The drawing under review shows one solid part. Ordinate dimensions are in mm from its lowest x, y, z. A direction names the side the tool comes from. Give positions to 0.01 mm unless a question says otherwise; leave off trailing zeros. Write each loop counter-clockwise with the first axis right and the second up, starting at its lowest first coordinate (ties: lowest second). Pieces come first, ordered by that corner, then holes.
Q1. We need section D-D (y = 16.75). Write out the cut boundary in (x, z).
Q2. Machinability: for the marked faces 1, 2, 3, 4 and 5, which of the approach directions +Z, -Z, +X, -X, +Y, -Y give a long, thin tool a straight path to every point of the face, cutting with its end or side? Answer none if there is none.
Q3. For line 1 (X direction, y = 4, z = 7.5); line 2 (Z direction, x = 37, y = 14); line 3 (Z direction, x = 5, y = 5.25), list the stretches that pass through material, from the lowest coordinate up.
Q4. We need section C-C (x = 6). Write out the cut boundary in (y, z).
Q5. We need section A-A (z = 17.5). Write out the cut boundary in (x, y).
Q6. Insertion check: P1, Ø5.5, axis at x = 36, z = 19, coming from the -Y side; P2, Ø5, axis at x = 7, z = 7.5, coming from the -Y side; P3, Ø1.5, axis at y = 2, z = 6, coming from the +X side; P4, Ø0.6, axis at y = 1, z = 15, coming from the +X side. Each pin has a flat end and moves straight along its axis. Give the tip position at first contact, or say it passes through.
Q7. We need section B-B (x = 37). Write out the cut boundary in (y, z).
Q8. Mouldability with a two-part tool opening along Z and no side actions: class the marked faces 6, 7, 8 and 9 as released by +Z, released by -Z, zero draft, split by the parting line, or undercut.
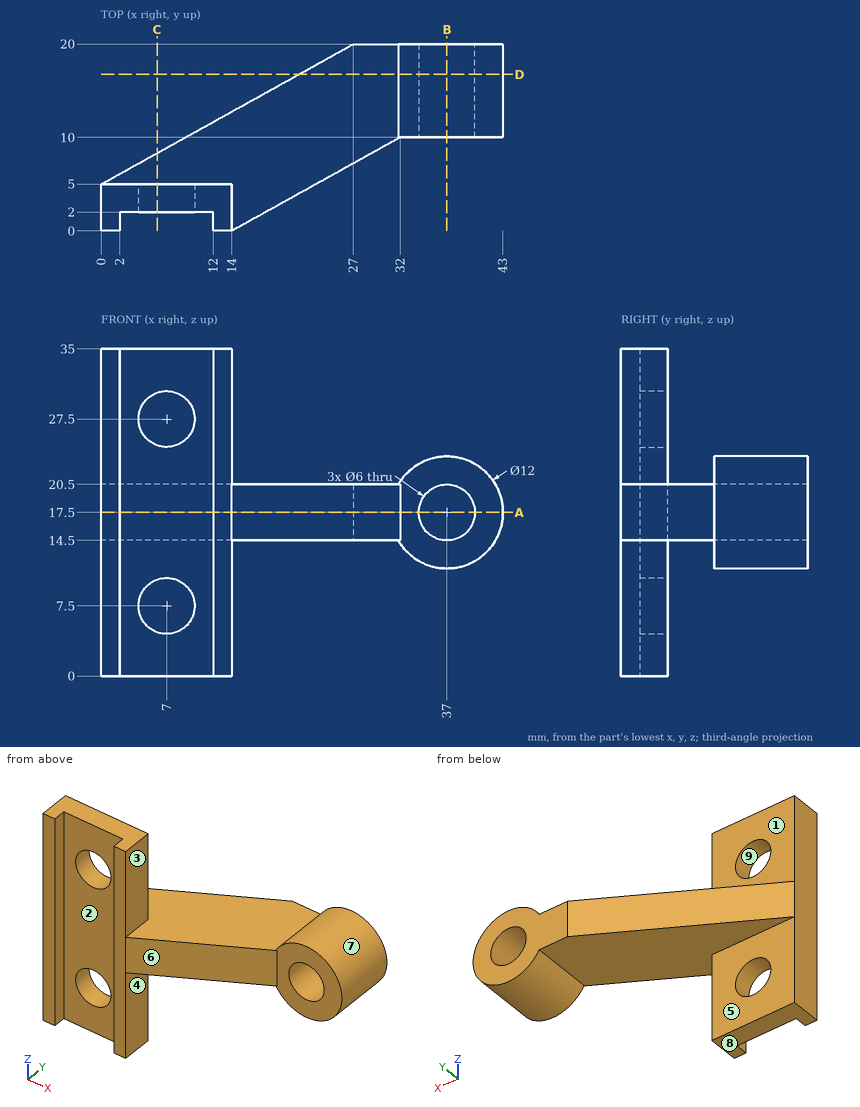
Computed:
1. outline: (21.15, 14.5) - (31.8, 14.5) arc R6 ccw (long way) to (31.8, 20.5) - (21.15, 20.5) - close; hole circle Ø6 at (37, 17.5)
2. face 1: +Z, +X, -X, +Y
2. face 2: +Z, -Z, -Y
2. face 3: +Z, +X, +Y, -Y
2. face 4: -Z, +X, +Y, -Y
2. face 5: -Z, +X, -X, +Y
3. line 1: x = 0 to 4, 10 to 14
3. line 2: z = 11.5 to 14.5, 20.5 to 23.5
3. line 3: z = 14.5 to 20.5
4. outline: (2, 0) - (5, 0) - (5, 4.67) - (2, 4.67) - close; (2, 10.33) - (5, 10.33) - (5, 14.5) - (8.33, 14.5) - (8.33, 20.5) - (5, 20.5) - (5, 24.67) - (2, 24.67) - close; (2, 30.33) - (5, 30.33) - (5, 35) - (2, 35) - close
5. outline: (0, 0) - (2, 0) - (2, 2) - (12, 2) - (12, 0) - (14, 0) - (32, 10) - (34, 10) - (34, 20) - (27, 20) - (0, 5) - close; (40, 10) - (43, 10) - (43, 20) - (40, 20) - close
6. P1: stops at y = 10
6. P2: passes through
6. P3: stops at x = 14
6. P4: stops at x = 16.34
7. outline: (10, 11.5) - (20, 11.5) - (20, 14.5) - (10, 14.5) - close; (10, 20.5) - (20, 20.5) - (20, 23.5) - (10, 23.5) - close
8. face 6: zero draft
8. face 7: split by the parting line
8. face 8: released by -Z
8. face 9: undercut
